```python
from build123d import *

# Parameters (mm, degrees)
F1_DEPTH = 2.5


with BuildPart() as f1:
    # F0 (on Right) → F1 (new body, symmetric)
    with BuildSketch(Plane.YZ):
        Polygon((-125, 25), (-125, 20), (-130, 20), (-130, 15), (-135, 15), (-135, 5), (-130, 5), (-130, -5), (-135, -5), (-135, -15), (-130, -15), (-130, -20), (-125, -20), (-125, -25), (-115, -25), (-115, -20), (-105, -20), (-105, -25), (-95, -25), (-95, -20), (-85, -20), (-85, -25), (-75, -25), (-75, -20), (-65, -20), (-65, -25), (-55, -25), (-55, -20), (-45, -20), (-45, -25), (-35, -25), (-35, -20), (-25, -20), (-25, -25), (-15, -25), (-15, -20), (-5, -20), (-5, -25), (5, -25), (5, -20), (15, -20), (15, -25), (25, -25), (25, -20), (35, -20), (35, -25), (45, -25), (45, -20), (55, -20), (55, -25), (65, -25), (65, -20), (75, -20), (75, -25), (85, -25), (85, -20), (95, -20), (95, -25), (105, -25), (105, -20), (115, -20), (115, -25), (125, -25), (125, -20), (135, -20), (135, -25), (145, -25), (145, -20), (155, -20), (155, -25), (165, -25), (165, -20), (175, -20), (175, -25), (185, -25), (185, -20), (195, -20), (195, -25), (205, -25), (205, -20), (215, -20), (215, -25), (225, -25), (225, -20), (235, -20), (235, -25), (245, -25), (245, -20), (250, -20), (250, -15), (255, -15), (255, -5), (250, -5), (250, 5), (255, 5), (255, 15), (250, 15), (250, 20), (245, 20), (245, 25), (235, 25), (235, 20), (225, 20), (225, 25), (215, 25), (215, 20), (205, 20), (205, 25), (195, 25), (195, 20), (185, 20), (185, 25), (175, 25), (175, 20), (165, 20), (165, 25), (155, 25), (155, 20), (145, 20), (145, 25), (135, 25), (135, 20), (125, 20), (125, 25), (115, 25), (115, 20), (105, 20), (105, 25), (95, 25), (95, 20), (85, 20), (85, 25), (75, 25), (75, 20), (65, 20), (65, 25), (55, 25), (55, 20), (45, 20), (45, 25), (35, 25), (35, 20), (25, 20), (25, 25), (15, 25), (15, 20), (5, 20), (5, 25), (-5, 25), (-5, 20), (-15, 20), (-15, 25), (-25, 25), (-25, 20), (-35, 20), (-35, 25), (-45, 25), (-45, 20), (-55, 20), (-55, 25), (-65, 25), (-65, 20), (-75, 20), (-75, 25), (-85, 25), (-85, 20), (-95, 20), (-95, 25), (-105, 25), (-105, 20), (-115, 20), (-115, 25), align=None)
    extrude(amount=F1_DEPTH, both=True)


solid = f1.part
```
The listing builds one solid part. Answer for the finished solid, in the listing's coordinates (mm). Coordinates: 2 decimals unless noted, no trailing zeros. Write each loop counter-clockwise with the first axis right and the second up, starting at its lowest first coordinate (ties: lowest second). Pieces come first, ordered by that corner, then holes. Notation, with made-up numbers: M 60,75 L 88,75 A7 ccw 88,85 Z; hole C 0,-32.5 d1. An arc over 180 degrees is marked long. Use a Markdown table: item, result. Add a question column.
1. Given P1, Ø1, axis at x = 2, z = -3, coming from the -Y side; P2, Ø2.5, axis at x = -1, y = -52, coming from the -Z side; P3, Ø1.5, axis at x = 0, z = -22.5, coming from the +Y side, each flat-ended and moving along its own axis, determine where each tip first touches the part or whether it passes through.
2. Section A-A (y = -69.5) is taken. Give the vertices of the cut face in (x, z).
3. Straight lines are drawn through the part: line 1 along Y through (x, z) = (-0.1, -0.5); line 2 along Z through (x, y) = (1.35, -27). For each, find the intervals that lie inside material, in ascending order. Write a range as [from, to].
Data:
| question | item | result |
|---|---|---|
| 1 | P1 | stops at y = -130 |
| 1 | P2 | stops at z = -20 |
| 1 | P3 | stops at y = 245 |
| 2 | outline | M -2.5,-20 L 2.5,-20 L 2.5,20 L -2.5,20 Z |
| 3 | line 1 | y = [-130, 250] |
| 3 | line 2 | z = [-20, 20] |
